```python
from build123d import *

# Parameters (mm, degrees)
SKETCH_3_R          = 65.2
EXTRUDE_2_DEPTH     = 5
SKETCH_4_R          = 63.2
SKETCH_4_R_2        = 62.2
CUT_EXTRUDE_3_DEPTH = 3
CUT_EXTRUDE_START   = -3
SKETCH_7_R          = 31
SKETCH_7_R_2        = 30
CUT_EXTRUDE_6_DEPTH = 3


# Read off the part's stored shape, not the designer's step: the shell step
with BuildPart() as part:
    # Sketch 1 → Revolve 1 (revolve)
    with BuildSketch(Plane.XY):
        Polygon((0, 0), (65.2, 0), (33, -200), (33, -205), (0, -205), align=None)
    revolve(axis=Axis((0, -205, 0), (0, 1, 0)))

    # Sketch 3 → Extrude 2 (add)
    with BuildSketch(Plane(origin=(0, 0, 0), x_dir=(1, 0, 0), z_dir=(0, 1, 0))):
        with Locations(Location((0, 0, 0), (0, 0, 180))):
            Circle(SKETCH_3_R)
    extrude(amount=EXTRUDE_2_DEPTH)

    # Shell 1 outline → Shell 1 (revolve, cut)
    with BuildSketch(Plane.XY):
        Polygon((0, 5), (0, -205), (30, -205), (30, -199.76004502), (62.2, 0.23995498), (62.2, 5), align=None)
    revolve(axis=Axis((0, 0, 0), (0, 1, 0)), mode=Mode.SUBTRACT)

    # Sketch 4 → Cut-Extrude 3 (cut)
    with BuildSketch(Plane(origin=(0, 5, 0), x_dir=(1, 0, 0), z_dir=(0, 1, 0))):
        with Locations(Location((0, 0, 0), (0, 0, 180))):
            Circle(SKETCH_4_R)
        with Locations(Location((0, 0, 0), (0, 0, 180))):
            Circle(SKETCH_4_R_2, mode=Mode.SUBTRACT)
    extrude(amount=-CUT_EXTRUDE_3_DEPTH, mode=Mode.SUBTRACT)

    # Sketch 7 → Cut-Extrude 6 (cut)
    with BuildSketch(Plane.XZ.offset(205).offset(CUT_EXTRUDE_START)):
        with Locations(Location((0, 0, 0), (0, 0, 270))):
            Circle(SKETCH_7_R)
        with Locations(Location((0, 0, 0), (0, 0, 270))):
            Circle(SKETCH_7_R_2, mode=Mode.SUBTRACT)
    extrude(amount=CUT_EXTRUDE_6_DEPTH, mode=Mode.SUBTRACT)


solid = part.part
```
Here's how the part is built. I have some questions about the finished solid (model axes, mm). A direction names the side the tool comes from. Round coordinates to 2 decimals unless told otherwise and drop trailing zeros. Loops run counter-clockwise (first coordinate to the right, second up) from the corner with the lowest first, then second, coordinate; pieces in that order, holes last.
1. For faces 1 (the face through (28, -202, 12)), 2 (the face through (27.712, -200.864, 11.49)), 3 (the face through (-42, 2, -47)), which set-ups out of +Z, -Z, +X, -X, +Y, -Y let a thin tool reach every point of the face, with its end or its side?
Answers:
face 1: -Y
face 2: +Y, -Y
face 3: +Y
2. Thinking about a two-plate mould opening in X: for faces 4 (the face through (-13.48, 1.13, 60.72)), 5 (the face through (51.74, 2.465, -39.673)), 6 (the face through (53.4, 5, 34.1)), which applies, released by +X, released by -X, zero draft, split by the parting line, or undercut?
Answers:
face 4: undercut
face 5: split by the parting line
face 6: zero draft
3. Suppose I cut it at D-D, the plane y = -165.5. Please give me the cut outline in (x, z), and give its area (3 significant figures).
Answers:
outline: circle Ø77.11 at (0, 0); hole circle Ø71.03 at (0, 0)
area: 707 mm2
4. If I drill on probe 1 along Z at (x, y) = (0, -201.2); probe 2 along X at (y, z) = (1.6, 0); probe 3 along Z at (x, y) = (0, 3), over which ranges is the centre line in solid material (lowest first)?
Answers:
probe 1: z = -33 to -30, 30 to 33
probe 2: x = -65.2 to -62.2, 62.2 to 65.2
probe 3: z = -65.2 to -63.2, 63.2 to 65.2
5. Suppose I cut it at C-C, the plane y = -131.5. Please give me the cut outline in (x, z).
Answers:
outline: circle Ø88.06 at (0, 0); hole circle Ø81.98 at (0, 0)
6. Suppose I cut it at B-B, the plane z = 0. Please give me the cut outline in (x, y).
Answers:
outline: (-65.2, 0) - (-33, -200) - (-33, -205) - (-31, -205) - (-31, -202) - (-30, -202) - (-30, -199.76) - (-62.2, 0.24) - (-62.2, 2) - (-63.2, 2) - (-63.2, 5) - (-65.2, 5) - close; (30, -202) - (31, -202) - (31, -205) - (33, -205) - (33, -200) - (65.2, 0) - (65.2, 5) - (63.2, 5) - (63.2, 2) - (62.2, 2) - (62.2, 0.24) - (30, -199.76) - close
7. Suppose I cut it at A-A, the plane x = 0. Please give me the cut outline in (y, z), and give its area (3 significant figures).
Answers:
outline: (-205, -33) - (-200, -33) - (0, -65.2) - (5, -65.2) - (5, -63.2) - (2, -63.2) - (2, -62.2) - (0.24, -62.2) - (-199.76, -30) - (-202, -30) - (-202, -31) - (-205, -31) - close; (-205, 31) - (-202, 31) - (-202, 30) - (-199.76, 30) - (0.24, 62.2) - (2, 62.2) - (2, 63.2) - (5, 63.2) - (5, 65.2) - (0, 65.2) - (-200, 33) - (-205, 33) - close
area: 1,260 mm2
8. Will these pins go through, and if not, where does the flat tip stop? pin 1 (12 mm diameter, centred on y = -87.5, z = 47, fed in from -X); pin 2 (12 mm diameter, centred on y = -74.5, z = 12, fed in from -X); pin 3 (6 mm diameter, centred on x = -49, y = -48.5, fed in from -Z); pin 4 (5 mm diameter, centred on x = 26, z = -22.5, fed in from -Y).
Answers:
pin 1: stops at x = -30.68
pin 2: stops at x = -53.33
pin 3: stops at z = -34.4
pin 4: stops at y = -205
